```python
from build123d import *

# Parameters (mm, degrees)
EXTRUDE1_REACH      = 31.416
EXTRUDE2_REACH      = 31.416
EXTRUDE2_END_RADIUS = 19.05
SKETCH3_R           = 2.4892
EXTRUDE3_REACH      = 31.416
EXTRUDE3_END_RADIUS = 19.05
SKETCH4_R           = 2.1717


with BuildPart() as part:
    # Sketch1 → Revolve1 (revolve)
    with BuildSketch(Plane(origin=(0, 0, 0), x_dir=(1, 0, 0), z_dir=(0, 1, 0)), mode=Mode.PRIVATE) as revolve1_sk:
        Polygon((7.9375, 11.811), (7.9375, 0), (9.525, 0), (9.525, 4.191), (19.05, 4.191), (19.05, 11.811), align=None)
    revolve(revolve1_sk.sketch.rotate(Axis((0, 0, -72.820126568), (0, 0, 1)), 180), axis=Axis((0, 0, -72.820126568), (0, 0, 1)))

    # Extrude1: up to this face of the body (flat: up to its plane)
    extrude1_end = Plane(part.part.faces().sort_by_distance((8.206907684, 0, 0))[0])
    # Sketch2 → Extrude1 (cut, up to the picked face)
    with BuildSketch(Plane(origin=(0, 0, -11.811), x_dir=(-1, 0, 0), z_dir=(0, 0, -1)), mode=Mode.PRIVATE) as extrude1_sk1:
        with BuildLine():
            Line((1.905, 9.8425), (1.905, 7.705509798))
            ThreePointArc((1.905, 7.705509798), (0, -7.9375), (-1.905, 7.705509798))
            Line((-1.905, 7.705509798), (-1.905, 9.8425))
            Line((-1.905, 9.8425), (1.905, 9.8425))
        make_face()
    extrude1_tool1 = split(extrude(extrude1_sk1.sketch, amount=-EXTRUDE1_REACH, mode=Mode.PRIVATE), bisect_by=extrude1_end, keep=Keep.BOTH, mode=Mode.PRIVATE)
    add(extrude1_tool1.solids().sort_by(Axis((0, 0.325226, -11.811), (0, 0, 1)))[0], mode=Mode.SUBTRACT)

    # Extrude2: up to this cylinder (the profile starts inside it)
    extrude2_end = Plane(origin=(0, 0, -8.001), z_dir=(0, 0, -1)) * Cylinder(EXTRUDE2_END_RADIUS, 101.932, mode=Mode.PRIVATE)
    # Sketch3 → Extrude2 (cut, up to the surface)
    with BuildSketch(Plane(origin=(0, 0, 0), x_dir=(1, 0, 0), z_dir=(0, 1, 0)), mode=Mode.PRIVATE) as extrude2_sk1:
        with Locations(Location((0, 8.001, 0), (0, 0, 90))):
            Circle(SKETCH3_R)
    extrude2_tool1 = extrude(extrude2_sk1.sketch, amount=EXTRUDE2_REACH, mode=Mode.PRIVATE) & extrude2_end
    add(extrude2_tool1.solids().sort_by_distance((0, 0, -8.001))[0], mode=Mode.SUBTRACT)

    # Extrude3: up to this cylinder (the profile starts inside it)
    extrude3_end = Plane(origin=(0, 0, -8.001), z_dir=(0, 0, -1)) * Cylinder(EXTRUDE3_END_RADIUS, 101.932, mode=Mode.PRIVATE)
    # Sketch4 → Extrude3 (cut, up to the surface)
    with BuildSketch(Plane(origin=(0, 0, 0), x_dir=(0, 0, -1), z_dir=(1, 0, 0)), mode=Mode.PRIVATE) as extrude3_sk1:
        with Locations(Location((8.001, 0, 0), (0, 0, 180))):
            Circle(SKETCH4_R)
    extrude3_tool1 = extrude(extrude3_sk1.sketch, amount=EXTRUDE3_REACH, mode=Mode.PRIVATE) & extrude3_end
    add(extrude3_tool1.solids().sort_by_distance((0, 0, -8.001))[0], mode=Mode.SUBTRACT)


solid = part.part
```
The model under review builds one solid part; all positions refer to its coordinate system, in mm. A direction names the side the tool comes from. Round coordinates to 2 decimals unless told otherwise and drop trailing zeros. Loops run counter-clockwise (first coordinate to the right, second up) from the corner with the lowest first, then second, coordinate; pieces in that order, holes last. Notation, with made-up numbers: M 52.5,-21 L 103.5,-21 A19 cw 103.5,-4 Z; hole C 41,81 d9. An arc over 180 degrees is marked long. Write item = value, one per line.
Item 1: Machinability: for faces 4 (the flat face through (2, -8, 0)), 5 (the cylindrical face through (-0.748, 13.215, -10.375)), 6 (the flat face through (-1.905, 9, -3)), 7 (the cylindrical face through (13.26, -1.83, -6.83)), which of the approach directions +Z, -Z, +X, -X, +Y, -Y give a long, thin tool a straight path to every point of the face, cutting with its end or side? Answer none if there is none.
Return value:
face_4 = +Z, +X, -X, +Y, -Y
face_5 = +Y
face_6 = +Z, -Z
face_7 = +X
Item 2: For line 1 (Y direction, x = 0, z = -5.75); line 2 (Y direction, x = 10.5, z = -10); line 3 (X direction, y = 12.5, z = -7), list the stretches that pass through material, from the lowest coordinate up. Write a range as [from, to].
Return value:
line_1 = [-19.05, -7.94]
line_2 = [-15.9, -0.85], [0.85, 15.9]
line_3 = [-14.38, -2.28], [2.28, 14.38]
Item 3: Insertion check: P1, Ø2, axis at x = 6.5, z = -2, coming from the +Y side; P2, Ø4, axis at x = 0, z = -8.001, coming from the +Y side; P3, Ø2.5, axis at x = 0.5, z = -5.5, coming from the -Y side. Each pin has a flat end and moves straight along its axis. Give the tip position at first contact, or say it passes through.
Return value:
P1 = 7.78
P2 = -7.68
P3 = -19.05
Item 4: Take a section at A-A on x = 0. State how many separate pieces and enclosed holes the cut face has, then the cut area to 3 significant figures.
Return value:
separate_pieces = 3
enclosed_holes = 0
area = 116 mm2
Item 5: Take a section at D-D on x = 14. Write out the cut boundary in (y, z).
Return value:
outline = M -12.92,-11.81 L 12.92,-11.81 L 12.92,-4.19 L -12.92,-4.19 Z; hole C 0,-8 d4.34
Item 6: The part is to be moulded in two halves that separate along Y. For faces 1 (the cylindrical face through (-0.392, -9.517, -2.125)), 2 (the cylindrical face through (-0.32, -7.93, -5.82)), 3 (the flat face through (4, -9, -4.191)), say which applies: released by +Y, released by -Y, zero draft, split by the parting line, or undercut.
Return value:
face_1 = split by the parting line
face_2 = undercut
face_3 = zero draft
